Geometry check sheet. Reference: the model listing, model coordinates, mm. A direction names the side the tool comes from. Round coordinates to 2 decimals unless told otherwise and drop trailing zeros. Write each loop counter-clockwise with the first axis right and the second up, starting at its lowest first coordinate (ties: lowest second). Pieces come first, ordered by that corner, then holes. Notation, with made-up numbers: M 22,-13.5 L 47,-13.5 A31 ccw 47,25.5 Z; hole C 15.5,-4.75 d11. An arc over 180 degrees is marked long. Use a Markdown table: item, result.
Autodesk Inventor part; units mm, degrees
ref_plane "YZ Plane" through (0, 0, 0) normal (1, 0, 0) x (0, 1, 0)
ref_plane "XZ Plane" through (0, 0, 0) normal (0, 1, 0) x (-1, 0, 0)
ref_plane "XY Plane" through (0, 0, 0) normal (0, 0, 1) x (1, 0, 0)
sketch "Sketch1" plane through (0, 0, 0) normal (0, 0, 1) x (1, 0, 0)
  line L0 (-16.4487, 14.1051) -> (-9.6381, 18.058)
  line L1 (-16.4487, 14.1051) -> (-18.8393, 18.2241)
  line L2 (-18.8393, 12.7176) -> (-23.6081, 15.4709)
  line L3 (-23.6081, 15.4709) -> (-23.6081, 20.9774)
  line L4 (-23.6081, 20.9774) -> (-18.8393, 23.7306)
  line L5 (-18.8393, 23.7306) -> (-14.0705, 20.9774)
  line L6 (-14.0705, 20.9774) -> (-14.0705, 15.4709)
  line L7 (-14.0705, 15.4709) -> (-18.8393, 12.7176)
  dimension "d5" = 4.7625
extrude "Extrusion1" add sketch "Sketch1" along normal blind 152.4
sketch "Sketch3" plane through (0, 0, 0) normal (0, 0, -1) x (-1, 0, 0)
  line L0 (23.6081, 15.4709) -> (18.8393, 12.7176)
  line L1 (18.8393, 12.7176) -> (18.8393, 18.2241)
  circle A0 centre (18.8393, 18.2241) radius 4.7688
  point P0 (0, 0)
extrude "Extrusion3" add sketch "Sketch3" along normal blind 12.7 contours A0
properties part number "Sanded Hex Rod"
Item 1: Cross-section at A-A, the plane z = 75.5. Record the cut outline in (x, y), and give its area (3 significant figures).
Outcome:
| item | result |
|---|---|
| outline | M -23.61,15.47 L -18.84,12.72 L -14.07,15.47 L -14.07,20.98 L -18.84,23.73 L -23.61,20.98 Z |
| area | 78.8 mm2 |
Item 2: Access from +Z, -Z, +X, -X, +Y, -Y to the whole of each face (thin tool, end or side, straight path). Record for faces 1 (the face through (-23.244, 20.051, -6.261)), 2 (the face through (-19, 18, -12.7)).
Outcome:
| item | result |
|---|---|
| face 1 | -Z |
| face 2 | -Z, +X, -X, +Y, -Y |
Item 3: Go/stop test with a flat-tipped pin: pin 1 (1 mm diameter, centred on x = -17.5, z = 99, fed in from +Y). Record where the tip stops, or that it passes through.
Outcome:
| item | result |
|---|---|
| pin 1 | stops at y = 23.25 |
Item 4: Material ranges on line 1 along X through (y, z) = (13.5, 74.5); line 2 along Y through (x, z) = (-15, 14.5); line 3 along X through (y, z) = (22, 93.5), recorded low to high. Write a range as from..to.
Outcome:
| item | result |
|---|---|
| line 1 | x = -20.19..-17.48 |
| line 2 | y = 14.93..21.51 |
| line 3 | x = -21.84..-15.84 |
